```python
from build123d import *

# Parameters (mm, degrees)
F0_R         = 10
F0_R_2       = 3
F0_R_3       = 7.5
F1_DEPTH     = 10
F2_W         = 42
F2_H         = 50
F2_R         = 7.5
F3_DEPTH     = 5
F4_T1_DEPTH  = 403.7
F4_T3_DEPTH  = 103.3
F4_T5_DEPTH  = 27
F4_T7_DEPTH  = 25
F4_T9_DEPTH  = 27
F4_T11_DEPTH = 9.5
F4_T13_DEPTH = 9.5
F4_T16_ANGLE = 66.8830141294
F4_T18_ANGLE = 66.8830141294
F4_T20_ANGLE = 66.8830141294
F4_T22_ANGLE = 66.8830141294
F4_T24_ANGLE = 90
F4_T26_ANGLE = 90
F4_T28_ANGLE = 90
F4_T30_ANGLE = 90


# Not quite as in the source:
# - a fillet or chamfer that OpenCascade refuses, or shapes differently, is made with other operations: its cross-section is extruded or revolved along the edge and cut away or added


with BuildPart() as f1:
    # F0 (on Front) → F1 (new body)
    with BuildSketch(Plane.XZ):
        with BuildLine():
            Line((0, -5), (0, 0))
            Line((0, 0), (0, 5))
            ThreePointArc((0, 5), (-27.9508497187, 11.5983005625), (-50, 30))
            Line((-50, 30), (-62, 30))
            Line((-62, 30), (-62, 28))
            ThreePointArc((-62, 28), (-62.8786796564, 25.8786796564), (-65, 25))
            Line((-65, 25), (-332, 25))
            Line((-332, 25), (-599, 25))
            ThreePointArc((-599, 25), (-601.1213203436, 25.8786796564), (-602, 28))
            Line((-602, 28), (-602, 30))
            Line((-602, 30), (-614, 30))
            ThreePointArc((-614, 30), (-636.0491502813, 11.5983005625), (-664, 5))
            Line((-664, 5), (-664, 0))
            Line((-664, 0), (-664, -5))
            ThreePointArc((-664, -5), (-636.0491502813, -11.5983005625), (-614, -30))
            Line((-614, -30), (-602, -30))
            Line((-602, -30), (-602, -28))
            ThreePointArc((-602, -28), (-601.1213203436, -25.8786796564), (-599, -25))
            Line((-599, -25), (-332, -25))
            Line((-332, -25), (-65, -25))
            ThreePointArc((-65, -25), (-62.8786796564, -25.8786796564), (-62, -28))
            Line((-62, -28), (-62, -30))
            Line((-62, -30), (-50, -30))
            ThreePointArc((-50, -30), (-27.9508497187, -11.5983005625), (0, -5))
        make_face()
        with Locations((-576.7, 0)):
            Circle(F0_R, mode=Mode.SUBTRACT)
        with Locations((-527.7, 0)):
            Circle(F0_R_2, mode=Mode.SUBTRACT)
        with Locations((-446.7, 0)):
            Circle(F0_R_2, mode=Mode.SUBTRACT)
        with Locations((-359.3, 0)):
            Circle(F0_R_2, mode=Mode.SUBTRACT)
        with Locations((-272.6, 0)):
            Circle(F0_R_2, mode=Mode.SUBTRACT)
        with Locations((-181.8, 0)):
            Circle(F0_R_3, mode=Mode.SUBTRACT)
    extrude(amount=F1_DEPTH)

    # F2 (on face) → F3 (cut)
    with BuildSketch(Plane.XZ.offset(10)):
        with Locations((-181.8, 0)):
            Rectangle(F2_W, F2_H)
        with Locations((-181.8, 0)):
            Circle(F2_R, mode=Mode.SUBTRACT)
    extrude(amount=-F3_DEPTH, mode=Mode.SUBTRACT)

    # F4: fillet of radius 3 on 18 edges, made by hand

    # F4_s2 → F4_t1 (cut)
    with BuildSketch(Plane.YZ.offset(-599)):
        with BuildLine():
            ThreePointArc((-10, 22), (-9.1213203436, 24.1213203436), (-7, 25))
            Line((-7, 25), (-10, 25))
            Line((-10, 25), (-10, 22))
        make_face()
        with BuildLine():
            ThreePointArc((-7, -25), (-9.1213203436, -24.1213203436), (-10, -22))
            Line((-10, -22), (-10, -25))
            Line((-10, -25), (-7, -25))
        make_face()
    extrude(amount=F4_T1_DEPTH, mode=Mode.SUBTRACT)

    # F4_s4 → F4_t3 (cut)
    with BuildSketch(Plane.YZ.offset(-168.3)):
        with BuildLine():
            ThreePointArc((-7, -25), (-9.1213203436, -24.1213203436), (-10, -22))
            Line((-10, -22), (-10, -25))
            Line((-10, -25), (-7, -25))
        make_face()
        with BuildLine():
            ThreePointArc((-10, 22), (-9.1213203436, 24.1213203436), (-7, 25))
            Line((-7, 25), (-10, 25))
            Line((-10, 25), (-10, 22))
        make_face()
    extrude(amount=F4_T3_DEPTH, mode=Mode.SUBTRACT)

    # F4_s6 → F4_t5 (cut)
    with BuildSketch(Plane.YZ.offset(-69.5)):
        with BuildLine():
            ThreePointArc((-10, -27), (-9.1213203436, -29.1213203436), (-7, -30))
            Line((-7, -30), (-10, -30))
            Line((-10, -30), (-10, -27))
        make_face()
        with BuildLine():
            ThreePointArc((-10, 27), (-9.1213203436, 29.1213203436), (-7, 30))
            Line((-7, 30), (-10, 30))
            Line((-10, 30), (-10, 27))
        make_face()
    extrude(amount=F4_T5_DEPTH, mode=Mode.SUBTRACT)

    # F4_s8 → F4_t7 (cut)
    with BuildSketch(Plane.XY.offset(-12.5)):
        with BuildLine():
            ThreePointArc((-3, -10), (-0.8786796564, -9.1213203436), (0, -7))
            Line((0, -7), (0, -10))
            Line((0, -10), (-3, -10))
        make_face()
        with BuildLine():
            ThreePointArc((-661, -10), (-663.1213203436, -9.1213203436), (-664, -7))
            Line((-664, -7), (-664, -10))
            Line((-664, -10), (-661, -10))
        make_face()
    extrude(amount=F4_T7_DEPTH, mode=Mode.SUBTRACT)

    # F4_s10 → F4_t9 (cut)
    with BuildSketch(Plane.YZ.offset(-621.5)):
        with BuildLine():
            ThreePointArc((-10, -27), (-9.1213203436, -29.1213203436), (-7, -30))
            Line((-7, -30), (-10, -30))
            Line((-10, -30), (-10, -27))
        make_face()
        with BuildLine():
            ThreePointArc((-10, 27), (-9.1213203436, 29.1213203436), (-7, 30))
            Line((-7, 30), (-10, 30))
            Line((-10, 30), (-10, 27))
        make_face()
    extrude(amount=F4_T9_DEPTH, mode=Mode.SUBTRACT)

    # F4_s12 → F4_t11 (cut)
    with BuildSketch(Plane.XY.offset(28)):
        with BuildLine():
            ThreePointArc((-605, -10), (-602.8786796564, -9.1213203436), (-602, -7))
            Line((-602, -7), (-602, -10))
            Line((-602, -10), (-605, -10))
        make_face()
        with BuildLine():
            ThreePointArc((-59, -10), (-61.1213203436, -9.1213203436), (-62, -7))
            Line((-62, -7), (-62, -10))
            Line((-62, -10), (-59, -10))
        make_face()
    extrude(amount=F4_T11_DEPTH, mode=Mode.SUBTRACT)

    # F4_s14 → F4_t13 (cut)
    with BuildSketch(Plane.XY.offset(-37.5)):
        with BuildLine():
            ThreePointArc((-605, -10), (-602.8786796564, -9.1213203436), (-602, -7))
            Line((-602, -7), (-602, -10))
            Line((-602, -10), (-605, -10))
        make_face()
        with BuildLine():
            ThreePointArc((-59, -10), (-61.1213203436, -9.1213203436), (-62, -7))
            Line((-62, -7), (-62, -10))
            Line((-62, -10), (-59, -10))
        make_face()
    extrude(amount=F4_T13_DEPTH, mode=Mode.SUBTRACT)

    # F4_s15 → F4_t16 (revolve, cut)
    with BuildSketch(Plane(origin=(-29.2244934886, 0, -50.6316906835), x_dir=(0, 1, 0), z_dir=(-0.4999008689, 0, -0.8660826296))):
        with BuildLine():
            ThreePointArc((-10, -31.7566913469), (-9.1213203436, -29.6353710033), (-7, -28.7566913469))
            Line((-7, -28.7566913469), (-10, -28.7566913469))
            Line((-10, -28.7566913469), (-10, -31.7566913469))
        make_face()
    revolve(axis=Axis((0, -10, -67.5), (0, 1, 0)), revolution_arc=F4_T16_ANGLE, mode=Mode.SUBTRACT)

    # F4_s17 → F4_t18 (revolve, cut)
    with BuildSketch(Plane(origin=(8.0235648794, 0, 0.9676128596), x_dir=(0, 1, 0), z_dir=(0.992806625, 0, 0.1197288826))):
        with BuildLine():
            ThreePointArc((-10, 1.5144471885), (-9.1213203436, 3.6357675321), (-7, 4.5144471885))
            Line((-7, 4.5144471885), (-10, 4.5144471885))
            Line((-10, 4.5144471885), (-10, 1.5144471885))
        make_face()
    revolve(axis=Axis((0, -10, 67.5), (0, 1, 0)), revolution_arc=F4_T18_ANGLE, mode=Mode.SUBTRACT)

    # F4_s19 → F4_t20 (revolve, cut)
    with BuildSketch(Plane(origin=(-662.5051213425, 0, -79.8957177472), x_dir=(0, 1, 0), z_dir=(-0.992806625, 0, -0.1197288826))):
        with BuildLine():
            ThreePointArc((-10, -77.9855308525), (-9.1213203436, -75.864210509), (-7, -74.9855308525))
            Line((-7, -74.9855308525), (-10, -74.9855308525))
            Line((-10, -74.9855308525), (-10, -77.9855308525))
        make_face()
    revolve(axis=Axis((-664, -10, -67.5), (0, 1, 0)), revolution_arc=F4_T20_ANGLE, mode=Mode.SUBTRACT)

    # F4_s21 → F4_t22 (revolve, cut)
    with BuildSketch(Plane(origin=(-136.7096900096, 0, -236.8507341524), x_dir=(0, 1, 0), z_dir=(0.4999008689, 0, 0.8660826296))):
        with BuildLine():
            ThreePointArc((-10, 543.3221746856), (-9.1213203436, 545.4434950292), (-7, 546.3221746856))
            Line((-7, 546.3221746856), (-10, 546.3221746856))
            Line((-10, 546.3221746856), (-10, 543.3221746856))
        make_face()
    revolve(axis=Axis((-664, -10, 67.5), (0, 1, 0)), revolution_arc=F4_T22_ANGLE, mode=Mode.SUBTRACT)

    # F4_s23 → F4_t24 (revolve, cut)
    with BuildSketch(Plane.YZ.offset(-65)):
        with BuildLine():
            ThreePointArc((-7, -25), (-9.1213203436, -24.1213203436), (-10, -22))
            Line((-10, -22), (-10, -25))
            Line((-10, -25), (-7, -25))
        make_face()
    revolve(axis=Axis((-65, -10, -28), (0, 1, 0)), revolution_arc=F4_T24_ANGLE, mode=Mode.SUBTRACT)

    # F4_s25 → F4_t26 (revolve, cut)
    with BuildSketch(Plane.XY.offset(28)):
        with BuildLine():
            ThreePointArc((-59, -10), (-61.1213203436, -9.1213203436), (-62, -7))
            Line((-62, -7), (-62, -10))
            Line((-62, -10), (-59, -10))
        make_face()
    revolve(axis=Axis((-65, -10, 28), (0, 1, 0)), revolution_arc=F4_T26_ANGLE, mode=Mode.SUBTRACT)

    # F4_s27 → F4_t28 (revolve, cut)
    with BuildSketch(Plane.XY.offset(-28)):
        with BuildLine():
            ThreePointArc((-605, -10), (-602.8786796564, -9.1213203436), (-602, -7))
            Line((-602, -7), (-602, -10))
            Line((-602, -10), (-605, -10))
        make_face()
    revolve(axis=Axis((-599, -10, -28), (0, 1, 0)), revolution_arc=F4_T28_ANGLE, mode=Mode.SUBTRACT)

    # F4_s29 → F4_t30 (revolve, cut)
    with BuildSketch(Plane.YZ.offset(-599)):
        with BuildLine():
            ThreePointArc((-10, 22), (-9.1213203436, 24.1213203436), (-7, 25))
            Line((-7, 25), (-10, 25))
            Line((-10, 25), (-10, 22))
        make_face()
    revolve(axis=Axis((-599, -10, 28), (0, 1, 0)), revolution_arc=F4_T30_ANGLE, mode=Mode.SUBTRACT)


solid = f1.part
```
Part model, mm, in its own coordinate system. Round coordinates to 2 decimals unless told otherwise and drop trailing zeros. Loops run counter-clockwise (first coordinate to the right, second up) from the corner with the lowest first, then second, coordinate; pieces in that order, holes last.
1. Two-plate mould, pull along X, no slides. Class faces 1 (the face through (-636.41, -3.45, -11.42)), 2 (the face through (-187, -5, 6)), 3 (the face through (-337, 0, 0)): pulls with the +X half, pulls with the -X half, needs draft (parallel to the pull), parting line crosses it, or undercut.
Solutions:
face 1: pulls with the -X half
face 2: undercut
face 3: needs draft
2. Slice it at B-B (x = -95.5). Give the cut face in (y, z).
Solutions:
outline: (-10, -22) arc R3 ccw to (-7, -25) - (0, -25) - (0, 25) - (-7, 25) arc R3 ccw to (-10, 22) - close
3. Slice it at A-A (x = -181.8). Give the cut face in (y, z), and give its area (3 significant figures).
Solutions:
outline: (-5, -25) - (0, -25) - (0, -7.5) - (-5, -7.5) - close; (-5, 7.5) - (0, 7.5) - (0, 25) - (-5, 25) - close
area: 175 mm2
4. Flat gauge pins, fed straight in: pin 1 (2 mm diameter, centred on y = -5, z = -28.5, fed in from -X); pin 2 (6 mm diameter, centred on y = -5, z = -16, fed in from +X); pin 3 (19.5 mm diameter, centred on x = -181.8, z = 0, fed in from -Y); pin 4 (3.5 mm diameter, centred on x = -446.7, z = 0, fed in from +Y). Where does each tip first touch, or does it go through?
Solutions:
pin 1: stops at x = -615.98
pin 2: stops at x = -30.59
pin 3: stops at y = -5
pin 4: passes through
5. Drill centre lines: line 1 along Z through (x, y) = (-181.8, -2.45); line 2 along Z through (x, y) = (-446.7, -4.75); line 3 along Z through (x, y) = (-520.5, -7.75). Where is each one in solid material? Low to high.
Solutions:
line 1: z = -25 to -7.5, 7.5 to 25
line 2: z = -25 to -3, 3 to 25
line 3: z = -24.9 to 24.9
6. Slice it at C-C (x = -576.7). Give the cut face in (y, z).
Solutions:
outline: (-10, -22) arc R3 ccw to (-7, -25) - (0, -25) - (0, -10) - (-10, -10) - close; (-10, 10) - (0, 10) - (0, 25) - (-7, 25) arc R3 ccw to (-10, 22) - close
